Model file for the job. Use its own axes, mm. A direction names the side the tool comes from. Round coordinates to 2 decimals unless told otherwise and drop trailing zeros. Loops run counter-clockwise (first coordinate to the right, second up) from the corner with the lowest first, then second, coordinate; pieces in that order, holes last.
Autodesk Inventor part; units mm, degrees
ref_plane "YZ Plane" through (0, 0, 0) normal (1, 0, 0) x (0, 1, 0)
ref_plane "XZ Plane" through (0, 0, 0) normal (0, 1, 0) x (-1, 0, 0)
ref_plane "XY Plane" through (0, 0, 0) normal (0, 0, 1) x (1, 0, 0)
sketch "Szkic1" plane through (0, 0, 0) normal (0, 1, 0) x (-1, 0, 0)
  line L0 (-4.5, -1.5) -> (4.5, -1.5)
  line L1 (4.5, -1.5) -> (4.5, 1.5)
  line L2 (4.5, 1.5) -> (-4.5, 1.5)
  line L3 (-4.5, 1.5) -> (-4.5, -1.5)
  line L4 (-4.5, -1.5) -> (4.5, 1.5) construction
  line L5 (4.5, -1.5) -> (-4.5, 1.5) construction
  point P0 (0, 0)
  dimension "d0" = 9
  dimension "d1" = 3
extrude "Wyciągnięcie proste1" add sketch "Szkic1" along normal blind 4
sketch "Szkic2" plane through (0, 0, 0) normal (0, -1, 0) x (1, 0, 0)
  line L0 (-5.5, -2.25) -> (5.5, -2.25)
  line L1 (5.5, -2.25) -> (5.5, 2.25)
  line L2 (5.5, 2.25) -> (-5.5, 2.25)
  line L3 (-5.5, 2.25) -> (-5.5, -2.25)
  line L4 (-5.5, -2.25) -> (5.5, 2.25) construction
  line L5 (5.5, -2.25) -> (-5.5, 2.25) construction
  point P0 (0, 0)
  dimension "d4" = 11
  dimension "d5" = 4.5
extrude "Wyciągnięcie proste2" add sketch "Szkic2" along normal blind 1
fillet "Zaokrąglenie1" radius 1 4 edges at (0, 4, 1.5) (-4.5, 4, 0) (0, 4, -1.5) (4.5, 4, 0)
properties part number "PRZYCISK"
Q1. Tool access for faces 1 (the face through (4.5, 1, 0)), 2 (the face through (0, 1, -1.5)), 3 (the face through (-4.5, 1, 0)), 4 (the face through (0, 1, 1.5)): list every direction of +Z, -Z, +X, -X, +Y, -Y with a clear straight run to the whole face (end or side of a thin tool).
Q2. Slice it at D-D on y = 3.2. Give the cut face in (x, z), plus the area to 3 significant figures.
Q3. Flat gauge pins, fed straight in: P1, Ø2.5, axis at y = 2, z = 0.5, coming from the +X side; P2, Ø2.5, axis at y = 1.5, z = 0, coming from the -X side; P3, Ø1.5, axis at x = 2, y = 1, coming from the +Z side. Where does each tip first touch, or does it go through?
Q4. Probe line 1 (Z direction, x = -1.5, y = 0.3); line 2 (Y direction, x = 5, z = 1.4); line 3 (X direction, y = 0.3, z = 0.6). List the from-to ranges inside material, lowest first.
Q5. Slice it at B-B on z = -0.35. Give the cut face in (x, y).
Q6. Slice it at A-A on x = 2.5. Give the cut face in (y, z).
Q7. Slice it at C-C on y = 1.4. Give the cut face in (x, z).
Reply:
1. face 1: +Z, -Z, +X, +Y
1. face 2: -Z, +X, -X, +Y
1. face 3: +Z, -Z, -X, +Y
1. face 4: +Z, +X, -X, +Y
2. outline: (-4.48, -1.48) - (4.48, -1.48) - (4.48, 1.48) - (-4.48, 1.48) - close
2. area: 26.5 mm2
3. P1: stops at x = 4.5
3. P2: stops at x = -4.5
3. P3: stops at z = 1.5
4. line 1: z = -1.5 to 1.5
4. line 2: y = -1 to 0
4. line 3: x = -4.5 to 4.5
5. outline: (-5.5, -1) - (5.5, -1) - (5.5, 0) - (4.5, 0) - (4.5, 3) arc R1 ccw to (3.5, 4) - (-3.5, 4) arc R1 ccw to (-4.5, 3) - (-4.5, 0) - (-5.5, 0) - close
6. outline: (-1, -2.25) - (0, -2.25) - (0, -1.5) - (3, -1.5) arc R1 ccw to (4, -0.5) - (4, 0.5) arc R1 ccw to (3, 1.5) - (0, 1.5) - (0, 2.25) - (-1, 2.25) - close
7. outline: (-4.5, -1.5) - (4.5, -1.5) - (4.5, 1.5) - (-4.5, 1.5) - close
